Could you check a few things on this drawing? It's one solid part, dimensions in mm from its lowest x, y, z. A direction names the side the tool comes from. Round coordinates to 2 decimals unless told otherwise and drop trailing zeros. Loops run counter-clockwise (first coordinate to the right, second up) from the corner with the lowest first, then second, coordinate; pieces in that order, holes last. Notation, with made-up numbers: M -20,-20.5 L 11,-20.5 A14 ccw 11,-6.5 Z; hole C 21.25,71 d2. An arc over 180 degrees is marked long. Answer as a JSON object with one key per item and string values.
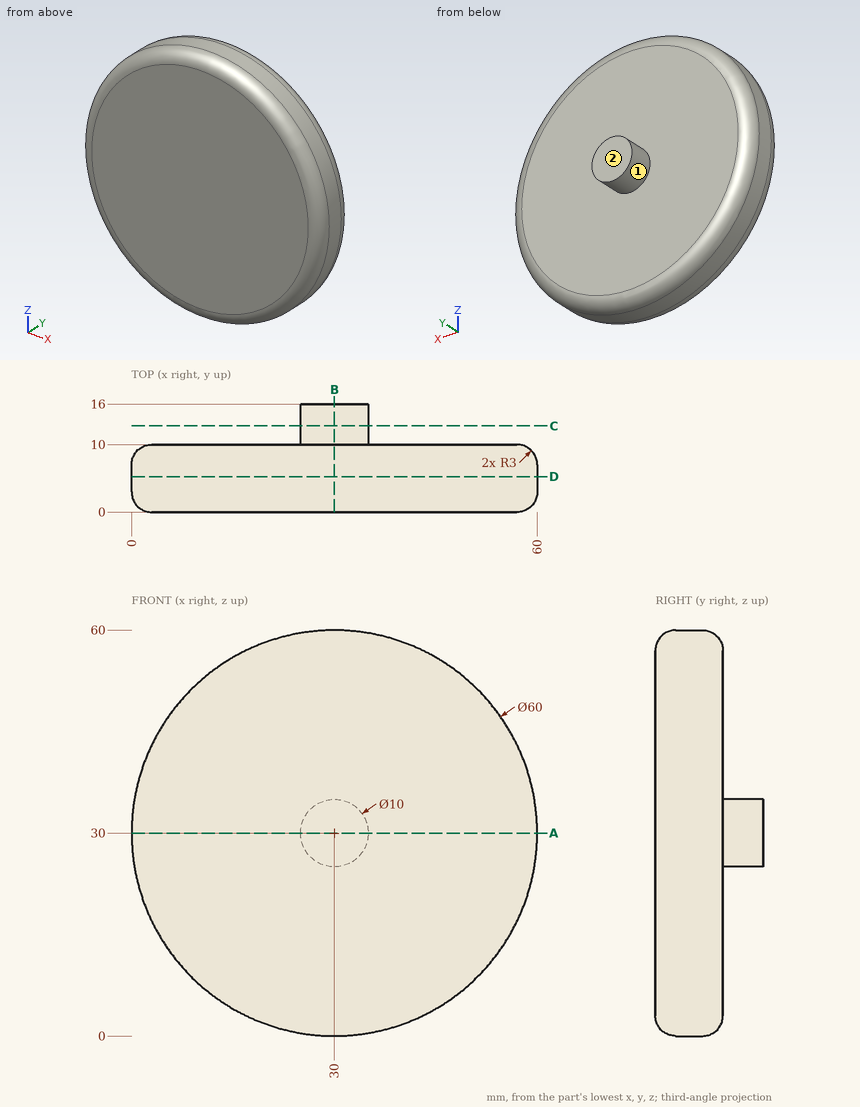
Item 1: Please list where these lines run through material, in increasing order: probe 1 along Y at (x, z) = (47.5, 10); probe 2 along Z at (x, y) = (22, 3.75); probe 3 along Z at (x, y) = (42, 7). Write a range as from..to.
Resolved:
{"probe 1": "0..10", "probe 2": "1.09..58.91", "probe 3": "2.5..57.5"}
Item 2: I want a section at C-C, the plane y = 12.75. Please give me the cut outline in (x, z), then the cut area to 3 significant figures.
Resolved:
{"outline": "C 30,30 d10", "area": "78.5 mm²"}
Item 3: I want a section at D-D, the plane y = 5.25. Please give me the cut outline in (x, z), then the cut area to 3 significant figures.
Resolved:
{"outline": "C 30,30 d60", "area": "2,830 mm²"}
Item 4: I want a section at A-A, the plane z = 30. Please give me the cut outline in (x, y), then the cut area to 3 significant figures.
Resolved:
{"outline": "M 0,3 A3 ccw 3,0 L 57,0 A3 ccw 60,3 L 60,7 A3 ccw 57,10 L 35,10 L 35,16 L 25,16 L 25,10 L 3,10 A3 ccw 0,7 Z", "area": "652 mm²"}
Item 5: I want a section at B-B, the plane x = 30. Please give me the cut outline in (y, z).
Resolved:
{"outline": "M 0,3 A3 ccw 3,0 L 7,0 A3 ccw 10,3 L 10,25 L 16,25 L 16,35 L 10,35 L 10,57 A3 ccw 7,60 L 3,60 A3 ccw 0,57 Z"}
Item 6: On a 3-axis mill with a long thin cutter (end or side, diameter ignored), from which of +Z, -Z, +X, -X, +Y, -Y can I reach the whole of each face in a straight line? I mean the marked faces 1 and 2. Say none if no direction works.
Resolved:
{"face 1": "+Y", "face 2": "+Z, -Z, +X, -X, +Y"}
Item 7: I'm going to push flat-ended pins straight in: pin 1 Ø12 at (x, z) = (49, 35.5) entering from +Y; pin 2 Ø1 at (x, y) = (34, 12.5) entering from +Z; pin 3 Ø8 at (x, y) = (37, 1.5) entering from +Z. Where does each tip first touch, or does it pass through?
Resolved:
{"pin 1": "y = 10", "pin 2": "z = 33.57", "pin 3": "z = 59.82"}
